Geometry check sheet. Reference: the model listing, model coordinates, mm. Give positions to 0.01 mm unless a question says otherwise; leave off trailing zeros. Write each loop counter-clockwise with the first axis right and the second up, starting at its lowest first coordinate (ties: lowest second). Pieces come first, ordered by that corner, then holes. Notation, with made-up numbers: (-36.5, 11) - (16.5, 11) arc R20 cw to (16.5, 47) - close; hole circle Ø7 at (41, 4.25). An arc over 180 degrees is marked (long way). Use a Markdown table: item, result.
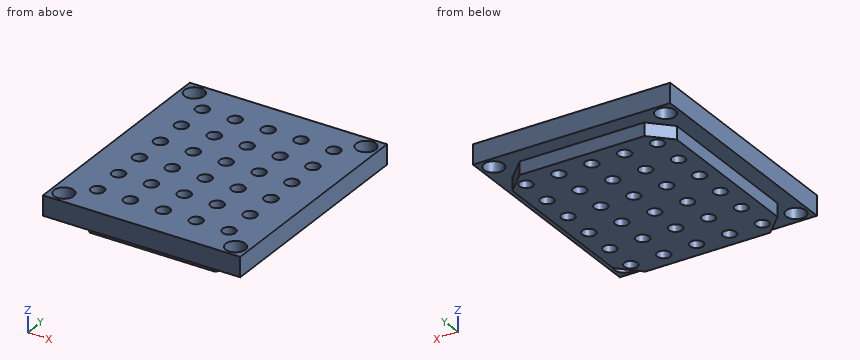
```python
from build123d import *

# Parameters (mm, degrees)
BOSS_EXTRU_4_DEPTH      = 2
ESQUISSE9_W             = 30
ESQUISSE9_H             = 35
BOSS_EXTRU_5_DEPTH      = 3
ESQUISSE7_R             = 1.5
ENL_V_MAT_EXTRU_8_DEPTH = 6
ESQUISSE10_R            = 1
ENL_V_MAT_EXTRU_9_DEPTH = 6


with BuildPart() as part:
    # Esquisse8 → Boss.-Extru.4 (new body)
    with BuildSketch(Plane.XY):
        Polygon((-9.5, 15), (9.5, 15), (12.5, 12), (12.5, -12), (9.5, -15), (-9.5, -15), (-12.5, -12), (-12.5, 12), align=None)
    extrude(amount=-BOSS_EXTRU_4_DEPTH)

    # Esquisse9 → Boss.-Extru.5 (add)
    with BuildSketch(Plane.XY):
        Rectangle(ESQUISSE9_W, ESQUISSE9_H)
    extrude(amount=BOSS_EXTRU_5_DEPTH)

    # Esquisse7 → Enlèv. mat.-Extru.8 (cut, through all)
    with BuildSketch(Plane.XY.offset(3)):
        with Locations((-13.055456352, 15.555456352)):
            Circle(ESQUISSE7_R)
        with Locations((-13.055456352, -15.555456352)):
            Circle(ESQUISSE7_R)
        with Locations((13.055456352, -15.555456352)):
            Circle(ESQUISSE7_R)
        with Locations((13.055456352, 15.555456352)):
            Circle(ESQUISSE7_R)
    extrude(amount=-ENL_V_MAT_EXTRU_8_DEPTH, mode=Mode.SUBTRACT)

    # Esquisse10 → Enlèv. mat.-Extru.9 (cut, through all)
    with BuildSketch(Plane.XY.offset(3)):
        with Locations((-9.890325409, 12.506661491)):
            Circle(ESQUISSE10_R)
        with Locations((-4.890325409, 12.506661491)):
            Circle(ESQUISSE10_R)
        with Locations((0.109674591, 12.506661491)):
            Circle(ESQUISSE10_R)
        with Locations((5.109674591, 12.506661491)):
            Circle(ESQUISSE10_R)
        with Locations((10.109674591, 12.506661491)):
            Circle(ESQUISSE10_R)
        with Locations((-4.890325409, 7.506661491)):
            Circle(ESQUISSE10_R)
        with Locations((0.109674591, 7.506661491)):
            Circle(ESQUISSE10_R)
        with Locations((5.109674591, 7.506661491)):
            Circle(ESQUISSE10_R)
        with Locations((10.109674591, 7.506661491)):
            Circle(ESQUISSE10_R)
        with Locations((-4.890325409, 2.506661491)):
            Circle(ESQUISSE10_R)
        with Locations((0.109674591, 2.506661491)):
            Circle(ESQUISSE10_R)
        with Locations((5.109674591, 2.506661491)):
            Circle(ESQUISSE10_R)
        with Locations((10.109674591, 2.506661491)):
            Circle(ESQUISSE10_R)
        with Locations((-4.890325409, -2.493338509)):
            Circle(ESQUISSE10_R)
        with Locations((0.109674591, -2.493338509)):
            Circle(ESQUISSE10_R)
        with Locations((5.109674591, -2.493338509)):
            Circle(ESQUISSE10_R)
        with Locations((10.109674591, -2.493338509)):
            Circle(ESQUISSE10_R)
        with Locations((-4.890325409, -7.493338509)):
            Circle(ESQUISSE10_R)
        with Locations((0.109674591, -7.493338509)):
            Circle(ESQUISSE10_R)
        with Locations((5.109674591, -7.493338509)):
            Circle(ESQUISSE10_R)
        with Locations((10.109674591, -7.493338509)):
            Circle(ESQUISSE10_R)
        with Locations((-4.890325409, -12.493338509)):
            Circle(ESQUISSE10_R)
        with Locations((0.109674591, -12.493338509)):
            Circle(ESQUISSE10_R)
        with Locations((5.109674591, -12.493338509)):
            Circle(ESQUISSE10_R)
        with Locations((10.109674591, -12.493338509)):
            Circle(ESQUISSE10_R)
        with Locations((-9.890325409, 7.506661491)):
            Circle(ESQUISSE10_R)
        with Locations((-9.890325409, 2.506661491)):
            Circle(ESQUISSE10_R)
        with Locations((-9.890325409, -2.493338509)):
            Circle(ESQUISSE10_R)
        with Locations((-9.890325409, -7.493338509)):
            Circle(ESQUISSE10_R)
        with Locations((-9.890325409, -12.493338509)):
            Circle(ESQUISSE10_R)
    extrude(amount=-ENL_V_MAT_EXTRU_9_DEPTH, mode=Mode.SUBTRACT)


solid = part.part
```
1) Depth check by flat-ended pin: P1, Ø1.8, axis at x = 0.11, y = -2.49, coming from the +Z side; P2, Ø0.6, axis at y = -2.5, z = -1, coming from the +X side; P3, Ø1.6, axis at x = 3, z = -1, coming from the +Y side. Enter the tip coordinate at first touch or a pass-through.
Working result:
| item | result |
|---|---|
| P1 | passes through |
| P2 | stops at x = 12.5 |
| P3 | stops at y = 15 |
2) Section check D-D on x = -10.25. Count the separate pieces of the cut face and the enclosed holes in it, then the cut area to 3 significant figures.
Working result:
| item | result |
|---|---|
| separate pieces | 7 |
| enclosed holes | 0 |
| area | 106 mm² |
3) Section check B-B on x = 2.75. Record the boundary of the cut face in (y, z), then the cut area to 3 significant figures.
Working result:
| item | result |
|---|---|
| outline | (-17.5, 0) - (-15, 0) - (-15, -2) - (15, -2) - (15, 0) - (17.5, 0) - (17.5, 3) - (-17.5, 3) - close |
| area | 165 mm² |
4) Material ranges on L1, parallel to X at y = 12.5, z = -0.15; L2, parallel to Y at x = 13, z = 0.8; L3, parallel to X at y = -2, z = -0.3, recorded low to high. Write a range as from..to.
Working result:
| item | result |
|---|---|
| L1 | x = -12..-10.89, -8.89..-5.89, -3.89..-0.89, 1.11..4.11, 6.11..9.11, 11.11..12 |
| L2 | y = -17.5..-17.05, -14.06..14.06, 17.05..17.5 |
| L3 | x = -12.5..-10.76, -9.02..-5.76, -4.02..-0.76, 0.98..4.24, 5.98..9.24, 10.98..12.5 |
5) Section check A-A on y = -7. Record the boundary of the cut face in (x, z), then the cut area to 3 significant figures.
Working result:
| item | result |
|---|---|
| outline | (-15, 0) - (-12.5, 0) - (-12.5, -2) - (-10.76, -2) - (-10.76, 3) - (-15, 3) - close; (-9.02, -2) - (-5.76, -2) - (-5.76, 3) - (-9.02, 3) - close; (-4.02, -2) - (-0.76, -2) - (-0.76, 3) - (-4.02, 3) - close; (0.98, -2) - (4.24, -2) - (4.24, 3) - (0.98, 3) - close; (5.98, -2) - (9.24, -2) - (9.24, 3) - (5.98, 3) - close; (10.98, -2) - (12.5, -2) - (12.5, 0) - (15, 0) - (15, 3) - (10.98, 3) - close |
| area | 96.5 mm² |
6) Section check C-C on y = 4. Record the boundary of the cut face in (x, z), then the cut area to 3 significant figures.
Working result:
| item | result |
|---|---|
| outline | (-15, 0) - (-12.5, 0) - (-12.5, -2) - (12.5, -2) - (12.5, 0) - (15, 0) - (15, 3) - (-15, 3) - close |
| area | 140 mm² |
